The listing builds one solid part. Answer for the finished solid, in the listing's coordinates (mm). Face numbers are marked on the shaded views. Round coordinates to 2 decimals unless told otherwise and drop trailing zeros. Loops run counter-clockwise (first coordinate to the right, second up) from the corner with the lowest first, then second, coordinate; pieces in that order, holes last. Notation, with made-up numbers: (7.5, -21) - (21.5, -21) arc R8 ccw to (21.5, -14) - close; hole circle Ø11 at (-32, 11.5). An arc over 180 degrees is marked (long way). One line per item, written item: value.
```python
from build123d import *

# Parameters (mm, degrees)
F0_W      = 89
F0_H      = 45
F1_DEPTH  = 5
F2_W      = 70
F2_H      = 39
F3_DEPTH  = 25
F4_W      = 85.5
F4_H      = 41.5
F5_DEPTH  = 3
F6_W      = 8
F6_H      = 8
F6_H_2    = 12
F7_DEPTH  = 3
F8_R      = 1
F9_DEPTH  = 25
F10_DEPTH = 25
F11_W     = 2.5
F11_H     = 2
F12_DEPTH = 25
F13_W     = 89
F13_H     = 3
F14_DEPTH = 25
F15_W     = 89
F15_H     = 9
F16_DEPTH = 1.5
F17_SIZE  = 1
F18_SIZE  = 1
F19_R     = 2
F20_R     = 0.5


with BuildPart() as f1:
    # F0 (on Top) → F1 (new body)
    with BuildSketch(Plane.XY):
        Rectangle(F0_W, F0_H)
    extrude(amount=F1_DEPTH)

    # F2 (on Top) → F3 (cut)
    with BuildSketch(Plane.XY):
        Rectangle(F2_W, F2_H)
    extrude(amount=F3_DEPTH, mode=Mode.SUBTRACT)

    # F4 (on Top) → F5 (cut)
    with BuildSketch(Plane.XY):
        Rectangle(F4_W, F4_H)
    extrude(amount=F5_DEPTH, mode=Mode.SUBTRACT)

    # F6 (on Top) → F7 (join)
    with BuildSketch(Plane.XY):
        with Locations((-40.5, 18.5)):
            Rectangle(F6_W, F6_H)
        with Locations((-40.5, -16.5)):
            Rectangle(F6_W, F6_H_2)
        with Locations((40.5, 18.5)):
            Rectangle(F6_W, F6_H)
        with Locations((40.5, -16.5)):
            Rectangle(F6_W, F6_H_2)
    extrude(amount=F7_DEPTH)

    # F8 (on Top) → F9 (cut)
    with BuildSketch(Plane.XY):
        with BuildLine():
            Line((39.25, -13.5), (41.75, -13.5))
            ThreePointArc((41.75, -13.5), (40.5, -12.25), (39.25, -13.5))
        make_face()
        with BuildLine():
            Line((41.75, -23.5), (41.75, -13.5))
            ThreePointArc((41.75, -13.5), (40.5, -14.75), (39.25, -13.5))
            Line((39.25, -13.5), (39.25, -23.5))
            Line((39.25, -23.5), (41.75, -23.5))
        make_face()
        with BuildLine():
            ThreePointArc((39.25, -13.5), (40.5, -14.75), (41.75, -13.5))
            Line((41.75, -13.5), (39.25, -13.5))
        make_face()
        with BuildLine():
            ThreePointArc((41.25, 18.5), (41.6180339887, 18.9409830056), (41.75, 19.5))
            ThreePointArc((41.75, 19.5), (39.9409830056, 20.6180339887), (39.75, 18.5))
            ThreePointArc((39.75, 18.5), (40.5, 18.75), (41.25, 18.5))
        make_face()
        with BuildLine():
            ThreePointArc((41.25, 18.5), (40.5, 18.75), (39.75, 18.5))
            ThreePointArc((39.75, 18.5), (40.5, 18.25), (41.25, 18.5))
        make_face()
        with BuildLine():
            ThreePointArc((41.25, 18.5), (40.5, 18.25), (39.75, 18.5))
            ThreePointArc((39.75, 18.5), (39.9409830056, 16.3819660113), (41.75, 17.5))
            ThreePointArc((41.75, 17.5), (41.6180339887, 18.0590169944), (41.25, 18.5))
        make_face()
        with BuildLine():
            Line((-41.75, -13.5), (-39.25, -13.5))
            ThreePointArc((-39.25, -13.5), (-40.5, -12.25), (-41.75, -13.5))
        make_face()
        with BuildLine():
            Line((-39.25, -23.5), (-39.25, -13.5))
            ThreePointArc((-39.25, -13.5), (-40.5, -14.75), (-41.75, -13.5))
            Line((-41.75, -13.5), (-41.75, -23.5))
            Line((-41.75, -23.5), (-39.25, -23.5))
        make_face()
        with BuildLine():
            ThreePointArc((-41.75, -13.5), (-40.5, -14.75), (-39.25, -13.5))
            Line((-39.25, -13.5), (-41.75, -13.5))
        make_face()
        with BuildLine():
            ThreePointArc((-39.75, 18.5), (-39.3819660113, 18.9409830056), (-39.25, 19.5))
            ThreePointArc((-39.25, 19.5), (-41.0590169944, 20.6180339887), (-41.25, 18.5))
            ThreePointArc((-41.25, 18.5), (-40.5, 18.75), (-39.75, 18.5))
        make_face()
        with BuildLine():
            ThreePointArc((-39.75, 18.5), (-40.5, 18.75), (-41.25, 18.5))
            ThreePointArc((-41.25, 18.5), (-40.5, 18.25), (-39.75, 18.5))
        make_face()
        with BuildLine():
            ThreePointArc((-39.75, 18.5), (-40.5, 18.25), (-41.25, 18.5))
            ThreePointArc((-41.25, 18.5), (-41.0590169944, 16.3819660113), (-39.25, 17.5))
            ThreePointArc((-39.25, 17.5), (-39.3819660113, 18.0590169944), (-39.75, 18.5))
        make_face()
        with Locations((-39, 0)):
            Circle(F8_R)
        with Locations((39, 0)):
            Circle(F8_R)
    extrude(amount=F9_DEPTH, mode=Mode.SUBTRACT)

    # F8 (on Top) → F10 (cut)
    with BuildSketch(Plane.XY):
        with BuildLine():
            Line((39.25, -13.5), (41.75, -13.5))
            ThreePointArc((41.75, -13.5), (40.5, -12.25), (39.25, -13.5))
        make_face()
        with BuildLine():
            Line((41.75, -23.5), (41.75, -13.5))
            ThreePointArc((41.75, -13.5), (40.5, -14.75), (39.25, -13.5))
            Line((39.25, -13.5), (39.25, -23.5))
            Line((39.25, -23.5), (41.75, -23.5))
        make_face()
        with BuildLine():
            ThreePointArc((39.25, -13.5), (40.5, -14.75), (41.75, -13.5))
            Line((41.75, -13.5), (39.25, -13.5))
        make_face()
        with BuildLine():
            ThreePointArc((41.25, 18.5), (41.6180339887, 18.9409830056), (41.75, 19.5))
            ThreePointArc((41.75, 19.5), (39.9409830056, 20.6180339887), (39.75, 18.5))
            ThreePointArc((39.75, 18.5), (40.5, 18.75), (41.25, 18.5))
        make_face()
        with BuildLine():
            ThreePointArc((41.25, 18.5), (40.5, 18.75), (39.75, 18.5))
            ThreePointArc((39.75, 18.5), (40.5, 18.25), (41.25, 18.5))
        make_face()
        with BuildLine():
            ThreePointArc((41.25, 18.5), (40.5, 18.25), (39.75, 18.5))
            ThreePointArc((39.75, 18.5), (39.9409830056, 16.3819660113), (41.75, 17.5))
            ThreePointArc((41.75, 17.5), (41.6180339887, 18.0590169944), (41.25, 18.5))
        make_face()
        with BuildLine():
            Line((-41.75, -13.5), (-39.25, -13.5))
            ThreePointArc((-39.25, -13.5), (-40.5, -12.25), (-41.75, -13.5))
        make_face()
        with BuildLine():
            Line((-39.25, -23.5), (-39.25, -13.5))
            ThreePointArc((-39.25, -13.5), (-40.5, -14.75), (-41.75, -13.5))
            Line((-41.75, -13.5), (-41.75, -23.5))
            Line((-41.75, -23.5), (-39.25, -23.5))
        make_face()
        with BuildLine():
            ThreePointArc((-41.75, -13.5), (-40.5, -14.75), (-39.25, -13.5))
            Line((-39.25, -13.5), (-41.75, -13.5))
        make_face()
        with BuildLine():
            ThreePointArc((-39.75, 18.5), (-39.3819660113, 18.9409830056), (-39.25, 19.5))
            ThreePointArc((-39.25, 19.5), (-41.0590169944, 20.6180339887), (-41.25, 18.5))
            ThreePointArc((-41.25, 18.5), (-40.5, 18.75), (-39.75, 18.5))
        make_face()
        with BuildLine():
            ThreePointArc((-39.75, 18.5), (-40.5, 18.75), (-41.25, 18.5))
            ThreePointArc((-41.25, 18.5), (-40.5, 18.25), (-39.75, 18.5))
        make_face()
        with BuildLine():
            ThreePointArc((-39.75, 18.5), (-40.5, 18.25), (-41.25, 18.5))
            ThreePointArc((-41.25, 18.5), (-41.0590169944, 16.3819660113), (-39.25, 17.5))
            ThreePointArc((-39.25, 17.5), (-39.3819660113, 18.0590169944), (-39.75, 18.5))
        make_face()
        with Locations((-39, 0)):
            Circle(F8_R)
        with Locations((39, 0)):
            Circle(F8_R)
    extrude(amount=F10_DEPTH, mode=Mode.SUBTRACT)

    # F11 (on face) → F12 (cut)
    with BuildSketch(Plane(origin=(0, 0, 0), x_dir=(1, 0, 0), z_dir=(0, 0, -1))):
        with Locations((-40.5, -18.5)):
            Rectangle(F11_W, F11_H)
        with Locations((40.5, -18.5)):
            Rectangle(F11_W, F11_H)
    extrude(amount=-F12_DEPTH, mode=Mode.SUBTRACT)

    # F13 (on face) → F14 (cut)
    with BuildSketch(Plane.XY.offset(5)):
        with Locations((0, -21)):
            Rectangle(F13_W, F13_H)
    extrude(amount=-F14_DEPTH, mode=Mode.SUBTRACT)

    # F15 (on face) → F16 (cut)
    with BuildSketch(Plane.XY.offset(5)):
        with Locations((0, -15)):
            Rectangle(F15_W, F15_H)
    extrude(amount=-F16_DEPTH, mode=Mode.SUBTRACT)

    # F17
    f17_edges = [f1.edges().sort_by_distance(p)[0] for p in [
        (41.75, 18.5, 5),
    ]]
    chamfer(f17_edges, length=F17_SIZE)

    # F18
    f18_edges = [f1.edges().sort_by_distance(p)[0] for p in [
        (-39.25, 18.5, 5),
    ]]
    chamfer(f18_edges, length=F18_SIZE)

    # F19
    f19_edges = [f1.edges().sort_by_distance(p)[0] for p in [
        (-44.5, 22.5, 2.5),
        (44.5, 22.5, 2.5),
        (35, 19.5, 4),
        (-35, 19.5, 4),
        (-36.5, 14.5, 1.5),
        (-36.5, 20.75, 1.5),
        (-42.75, 14.5, 1.5),
        (-42.75, -10.5, 1.5),
        (-36.5, -10.5, 1.5),
        (36.5, 20.75, 1.5),
        (36.5, 14.5, 1.5),
        (42.75, 14.5, 1.5),
        (42.75, -10.5, 1.5),
        (36.5, -10.5, 1.5),
    ]]
    fillet(f19_edges, radius=F19_R)

    # F20
    f20_edges = [f1.edges().sort_by_distance(p)[0] for p in [
        (0, 22.5, 5),
        (-39.75, -10.5, 5),
        (39.75, -10.5, 5),
        (35, 3.5, 5),
    ]]
    fillet(f20_edges, radius=F20_R)


solid = f1.part
```
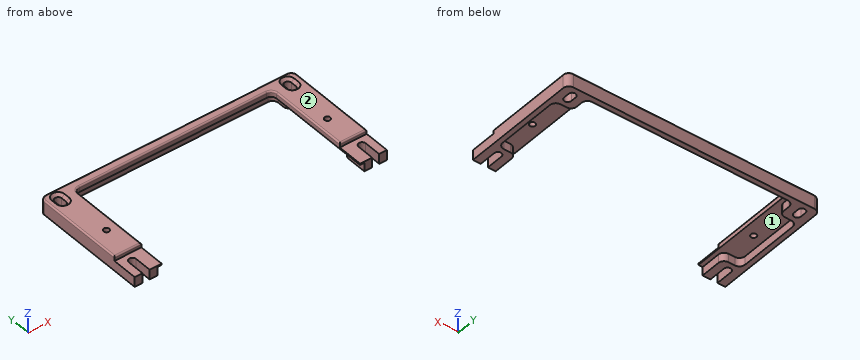
1) A cutting plane is placed at B-B on x = -27. Give the vertices of the cut face in (y, z).
Final values:
outline: (19.5, 3) - (20.75, 3) - (20.75, 0) - (22.5, 0) - (22.5, 4.5) arc R0.5 ccw to (22, 5) - (20, 5) arc R0.5 ccw to (19.5, 4.5) - close
2) Each of these flat-tipped pins is pushed along its axis until it touches: pin 1 Ø2.5 at (x, y) = (-39, -17) entering from +Z; pin 2 Ø8 at (x, y) = (-34, -8) entering from -Z; pin 3 Ø0.7 at (x, z) = (-39.5, 1.5) entering from -Y; pin 4 Ø2 at (x, z) = (-11, 2.5) entering from -Y. Where does it stop, or does it pass through?
Final values:
pin 1: z = 3.5
pin 2: z = 3
pin 3: y = -19.5
pin 4: y = 19.5
3) A cutting plane is placed at C-C on z = 0.85. Give the number of separate pieces and of enclosed holes in the cut face, and give its area (3 significant figures).
Final values:
separate pieces: 1
enclosed holes: 2
area: 433 mm2
4) For a pull along X with two mould halves and no side action, classify the marked faces 1 and 2 as released by +X, released by -X, zero draft, split by the parting line, or undercut.
Final values:
face 1: undercut
face 2: zero draft
5) Consider L1, parallel to X at y = 0, z = 3.85; L2, parallel to Y at x = 39, z = 4.55; L3, parallel to X at y = -10, z = 3.85. Determine where each line is inside the solid, lowest interval first.
Final values:
L1: -44.5 to -40, -38 to -35, 35 to 38, 40 to 44.5
L2: -10.5 to -1, 1 to 16.51, 20.49 to 22.5
L3: -44.5 to -35, 35 to 44.5
6) A cutting plane is placed at A-A on y = 10.5. Give the vertices of the cut face in (x, z), and give its area (3 significant figures).
Final values:
outline: (-44.5, 0) - (-42.75, 0) - (-42.75, 3) - (-35, 3) - (-35, 4.5) arc R0.5 ccw to (-35.5, 5) - (-44, 5) arc R0.5 ccw to (-44.5, 4.5) - close; (35, 3) - (42.75, 3) - (42.75, 0) - (44.5, 0) - (44.5, 4.5) arc R0.5 ccw to (44, 5) - (35.5, 5) arc R0.5 ccw to (35, 4.5) - close
area: 48.3 mm2
